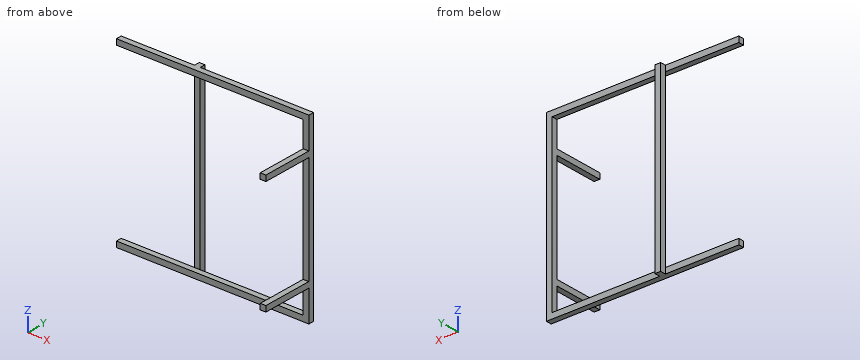
from build123d import *

# Parameters (mm, degrees)
SKETCH_1_W          = 380.612698372
SKETCH_1_H          = 600
EXTRUDE_1_DEPTH     = 20
SKETCH1_W           = 20
SKETCH1_H           = 640
BOSS_EXTRUDE1_DEPTH = 20
SKETCH2_W           = 20
SKETCH2_H           = 600
CUT_EXTRUDE1_DEPTH  = 20
SKETCH3_W           = 20
SKETCH3_H           = 20
BOSS_EXTRUDE2_DEPTH = 180


with BuildPart() as part:
    # 草图1 → 凸台-拉伸1 (new body)
    with BuildSketch(Plane(origin=(0, 0, 0), x_dir=(1, 0, 0), z_dir=(0, 1, 0))):
        Polygon((-329.38787024, -472.094950635), (-329.38787024, -492.094950635), (350.61212976, -492.094950635), (350.61212976, 147.905049365), (-329.38787024, 147.905049365), (-329.38787024, 127.905049365), (-70.000568612, 127.905049365), (-70.000568612, -472.094950635), align=None)
        with Locations((140.305780574, -172.094950635)):
            Rectangle(SKETCH_1_W, SKETCH_1_H, mode=Mode.SUBTRACT)
    extrude(amount=EXTRUDE_1_DEPTH)

    # Sketch1 → Boss-Extrude1 (add)
    with BuildSketch(Plane(origin=(0, 20, 0), x_dir=(1, 0, 0), z_dir=(0, 1, 0))):
        with Locations((-60.000568612, -172.094950635)):
            Rectangle(SKETCH1_W, SKETCH1_H)
    extrude(amount=BOSS_EXTRUDE1_DEPTH)

    # Sketch2 → Cut-Extrude1 (cut)
    with BuildSketch(Plane.XZ):
        with Locations((-60.000568612, 172.094950635)):
            Rectangle(SKETCH2_W, SKETCH2_H)
    extrude(amount=-CUT_EXTRUDE1_DEPTH, mode=Mode.SUBTRACT)

    # Sketch3 → Boss-Extrude2 (add)
    with BuildSketch(Plane.XZ):
        with Locations((340.61212976, 372.094950635)):
            Rectangle(SKETCH3_W, SKETCH3_H)
        with Locations((340.61212976, -27.905049365)):
            Rectangle(SKETCH3_W, SKETCH3_H)
    extrude(amount=BOSS_EXTRUDE2_DEPTH)


solid = part.part
Verification items for the finished model (mm, model axes). Give positions to 0.01 mm unless a question says otherwise; leave off trailing zeros. Loops run counter-clockwise (first coordinate to the right, second up) from the corner with the lowest first, then second, coordinate; pieces in that order, holes last. Notation, with made-up numbers: (-33.5, 69.25) - (-5.5, 69.25) arc R24 cw to (-5.5, 90.25) - close; hole circle Ø6 at (78, -17.75). An arc over 180 degrees is marked (long way). Write each question's results on one line, items separated by ' | '.
1) Sectioned sample at A-A on x = -248.5. Record the boundary of the cut face in (y, z).
Solution:
outline: (0, -147.91) - (20, -147.91) - (20, -127.91) - (0, -127.91) - close; (0, 472.09) - (20, 472.09) - (20, 492.09) - (0, 492.09) - close
2) Material ranges on L1, parallel to X at y = 5, z = 343.5; L2, parallel to Z at x = 280.5, y = 15; L3, parallel to X at y = 21, z = 40.5, recorded low to high. Write a range as from..to.
Solution:
L1: 330.61..350.61 | L2: -147.91..-127.91, 472.09..492.09 | L3: -70..-50
3) Sectioned sample at B-B on y = -78.5. Record the boundary of the cut face in (x, z).
Solution:
outline: (330.61, -37.91) - (350.61, -37.91) - (350.61, -17.91) - (330.61, -17.91) - close; (330.61, 362.09) - (350.61, 362.09) - (350.61, 382.09) - (330.61, 382.09) - close
4) Depth check by flat-ended pin: P1, Ø16, axis at x = -204.5, z = 479.5, coming from the +Y side; P2, Ø10, axis at x = 337.5, y = -63.5, coming from the +Z side; P3, Ø10, axis at y = 30.5, z = 242.5, coming from the -X side. Enter the tip coordinate at first touch or a pass-through.
Solution:
P1: y = 20 | P2: z = 382.09 | P3: x = -70
